The drawing under review shows one solid part. Ordinate dimensions are in mm from its lowest x, y, z. Coordinates: 2 decimals unless noted, no trailing zeros. Write each loop counter-clockwise with the first axis right and the second up, starting at its lowest first coordinate (ties: lowest second). Pieces come first, ordered by that corner, then holes. Notation, with made-up numbers: (61, -33) - (78, -33) arc R13 cw to (78, -10) - close; hole circle Ø10 at (-25, -22). An arc over 180 degrees is marked (long way). Put each result on its own line as item: value. Start each with the question number.
Item 1: Consider section B-B on z = 25. Give the boundary of the cut face in (x, y), then the cut area to 3 significant figures.
Item 2: Consider section C-C on x = 39.5. Give the boundary of the cut face in (y, z).
Item 3: Consider section A-A on y = 20. Give the boundary of the cut face in (x, z).
Item 4: To check wall thickness, follow L1, parallel to Y at x = 22, z = 41; L2, parallel to X at y = 17, z = 40; L3, parallel to Z at x = 28, y = 13.5. State the ranges of each line that lie inside material, in increasing order. Write a range as [from, to].
Item 5: For pin 1 (17.5 mm diameter, centred on y = 21.844, z = 21.844, fed in from +X), flat-tipped, find the tip position at first contact; note if it passes through.
Item 6: Mouldability with a two-part tool opening along X and no side actions: class the marked faces 1, 2, 3 and 4 as pulls with the +X half, pulls with the -X half, needs draft (parallel to the pull), parting line crosses it, or undercut.
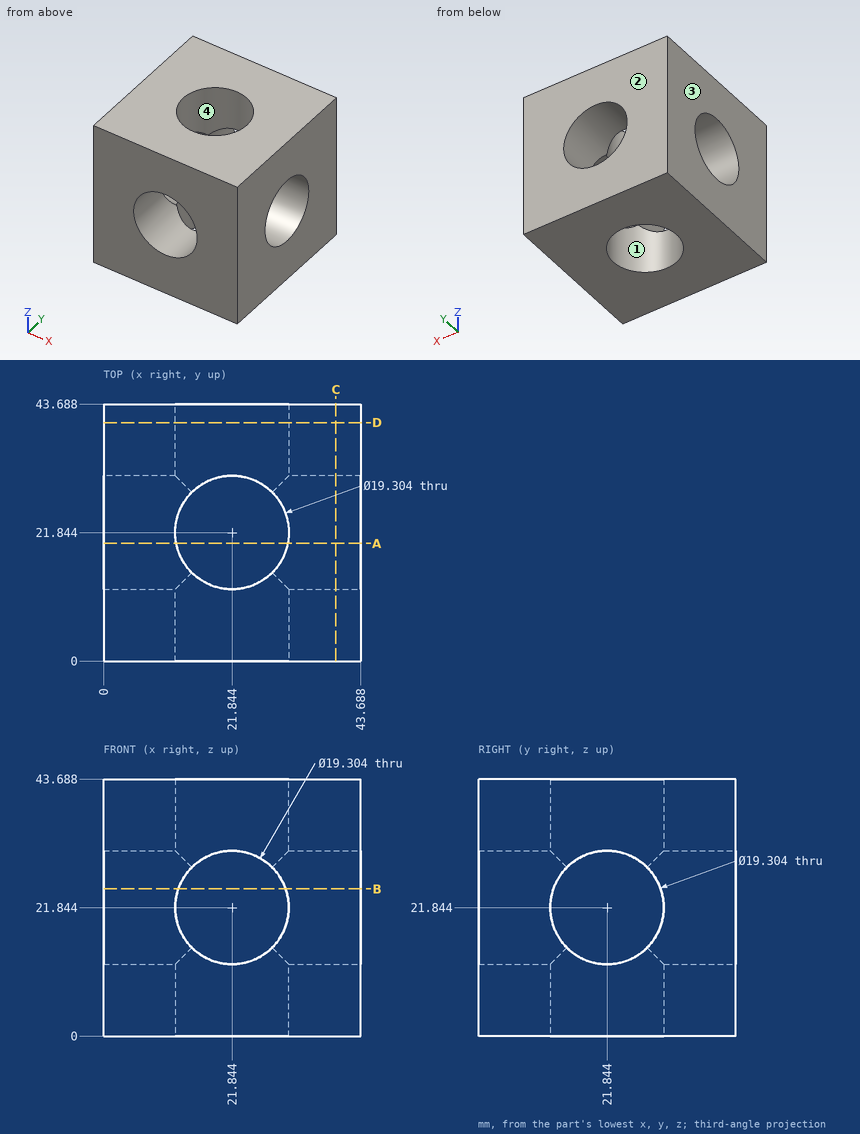
Report:
1. outline: (0, 0) - (12.72, 0) - (12.72, 12.72) - (0, 12.72) - close; (0, 30.97) - (12.72, 30.97) - (12.72, 43.69) - (0, 43.69) - close; (30.97, 0) - (43.69, 0) - (43.69, 12.72) - (30.97, 12.72) - close; (30.97, 30.97) - (43.69, 30.97) - (43.69, 43.69) - (30.97, 43.69) - close
1. area: 647 mm²
2. outline: (0, 0) - (43.69, 0) - (43.69, 43.69) - (0, 43.69) - close; hole circle Ø19.3 at (21.84, 21.84)
3. outline: (0, 0) - (12.37, 0) - (12.37, 12.37) - (0, 12.37) - close; (0, 31.32) - (12.37, 31.32) - (12.37, 43.69) - (0, 43.69) - close; (31.32, 0) - (43.69, 0) - (43.69, 12.37) - (31.32, 12.37) - close; (31.32, 31.32) - (43.69, 31.32) - (43.69, 43.69) - (31.32, 43.69) - close
4. L1: [0, 12.19], [31.49, 43.69]
4. L2: [0, 13.5], [30.19, 43.69]
4. L3: [0, 14.41], [29.28, 43.69]
5. pin 1: through
6. face 1: undercut
6. face 2: needs draft
6. face 3: pulls with the -X half
6. face 4: undercut
